from build123d import *

# Parameters (mm, degrees)
EXTRUDE_1_DEPTH     = 32
EXTRUDE_2_DEPTH     = 18
CUT_EXTRUDE_1_DEPTH = 204.283053893
SKETCH_5_W          = 110.763550328
SKETCH_5_H          = 22
CUT_EXTRUDE_2_DEPTH = 6
CUT_EXTRUDE_3_DEPTH = 36
CUT_EXTRUDE_4_DEPTH = 9
SKETCH_7_R          = 6.5
CUT_EXTRUDE_5_DEPTH = 181.357330689
SKETCH_8_W          = 38
SKETCH_8_H          = 7
EXTRUDE_3_DEPTH     = 30.5
EXTRUDE_START       = 14.5
SKETCH_8_3_R        = 9.5
EXTRUDE_4_DEPTH     = 16


with BuildPart() as part:
    # Sketch 1 → Extrude 1 (new, symmetric)
    with BuildSketch(Plane.XY):
        Polygon((0, 0), (-45, 77.942286341), (-28.545517328, 87.442286341), (8.758035362, 22.830637779), (140, 22.830637779), (140, 0), align=None)
    extrude(amount=EXTRUDE_1_DEPTH, both=True)

    # Sketch 2 → Extrude 2 (add)
    with BuildSketch(Plane(origin=(-45, 77.942286341, 0), x_dir=(0.8660254037844364, 0.5000000000000041, 0), z_dir=(-0.500000000000004, 0.8660254037844363, 0))):
        with BuildLine():
            Line((19, 32), (19, -32))
            Line((19, -32), (51, -32))
            ThreePointArc((51, -32), (83, 0), (51, 32))
            Line((51, 32), (19, 32))
        make_face()
    extrude(amount=-EXTRUDE_2_DEPTH)

    # Sketch 4 → Cut-Extrude 1 (cut, through all)
    with BuildSketch(Plane(origin=(-45, 77.942286341, 0), x_dir=(0.8660254037844364, 0.5000000000000041, 0), z_dir=(-0.500000000000004, 0.8660254037844363, 0))):
        Polygon((0, 21), (6, 17.535898385), (6, -17.535898385), (0, -21), align=None)
    extrude(amount=-CUT_EXTRUDE_1_DEPTH, mode=Mode.SUBTRACT)

    # Sketch 5 → Cut-Extrude 2 (cut)
    with BuildSketch(Plane(origin=(-45, 77.942286341, 0), x_dir=(0.8660254037844364, 0.5000000000000041, 0), z_dir=(-0.500000000000004, 0.8660254037844363, 0))):
        with Locations((41.909126347, 0)):
            Rectangle(SKETCH_5_W, SKETCH_5_H)
    extrude(amount=-CUT_EXTRUDE_2_DEPTH, mode=Mode.SUBTRACT)

    # Sketch 6 → Cut-Extrude 3 (cut)
    with BuildSketch(Plane(origin=(-45, 77.942286341, 0), x_dir=(0.8660254037844364, 0.5000000000000041, 0), z_dir=(-0.500000000000004, 0.8660254037844363, 0))):
        with BuildLine():
            ThreePointArc((41.5, 0), (51, -9.5), (60.5, 0))
            Line((60.5, 0), (41.5, 0))
        make_face()
        with BuildLine():
            Line((41.5, 0), (60.5, 0))
            ThreePointArc((60.5, 0), (51, 9.5), (41.5, 0))
        make_face()
    extrude(amount=-CUT_EXTRUDE_3_DEPTH, mode=Mode.SUBTRACT)

    # Sketch 6_3 → Cut-Extrude 4 (cut)
    with BuildSketch(Plane(origin=(-45, 77.942286341, 0), x_dir=(0.8660254037844364, 0.5000000000000041, 0), z_dir=(-0.500000000000004, 0.8660254037844363, 0))):
        with BuildLine():
            ThreePointArc((41.5, 0), (51, -9.5), (60.5, 0))
            Line((60.5, 0), (41.5, 0))
        make_face()
        with BuildLine():
            Line((41.5, 0), (60.5, 0))
            ThreePointArc((60.5, 0), (51, 9.5), (41.5, 0))
        make_face()
        with BuildLine():
            ThreePointArc((41.5, 0), (51, 9.5), (60.5, 0))
            Line((60.5, 0), (67, 0))
            ThreePointArc((67, 0), (65.8644408, 5.92016889), (62.618950039, 11))
            Line((62.618950039, 11), (39.381049961, 11))
            ThreePointArc((39.381049961, 11), (36.1355592, 5.92016889), (35, 0))
            Line((35, 0), (41.5, 0))
        make_face()
        with BuildLine():
            Line((39.381049961, 11), (62.618950039, 11))
            ThreePointArc((62.618950039, 11), (51, 16), (39.381049961, 11))
        make_face()
        with BuildLine():
            Line((67, 0), (60.5, 0))
            ThreePointArc((60.5, 0), (51, -9.5), (41.5, 0))
            Line((41.5, 0), (35, 0))
            ThreePointArc((35, 0), (51, -16), (67, 0))
        make_face()
    extrude(amount=-CUT_EXTRUDE_4_DEPTH, mode=Mode.SUBTRACT)

    # Sketch 7 → Cut-Extrude 5 (cut, through all)
    with BuildSketch(Plane(origin=(5.196152423, 3, 0), x_dir=(0, 0, 1), z_dir=(-0.8660254037844365, -0.500000000000004, 0))):
        with Locations(Location((0, 56, 0), (0, 0, 270))):
            Circle(SKETCH_7_R)
        with Locations(Location((0, 27, 0), (0, 0, 270))):
            Circle(SKETCH_7_R)
    extrude(amount=-CUT_EXTRUDE_5_DEPTH, mode=Mode.SUBTRACT)

    # Sketch 8 → Extrude 3 (add, symmetric)
    with BuildSketch(Plane(origin=(89.5, 0, 0), x_dir=(0, 0, -1), z_dir=(1, 0, 0))):
        with Locations((0, 26.330637779)):
            Rectangle(SKETCH_8_W, SKETCH_8_H)
    extrude(amount=EXTRUDE_3_DEPTH, both=True)

    # Sketch 8_3 → Extrude 4 (add)
    with BuildSketch(Plane(origin=(89.5, 0, 0), x_dir=(0, 0, -1), z_dir=(1, 0, 0)).offset(EXTRUDE_START)):
        with BuildLine():
            Line((-19, 54.830637779), (-19, 29.830637779))
            Line((-19, 29.830637779), (19, 29.830637779))
            Line((19, 29.830637779), (19, 54.830637779))
            ThreePointArc((19, 54.830637779), (0, 73.830637779), (-19, 54.830637779))
        make_face()
        with Locations((0, 54.830637779)):
            Circle(SKETCH_8_3_R, mode=Mode.SUBTRACT)
    extrude_4 = extrude(amount=EXTRUDE_4_DEPTH)

    # Mirror 1: Extrude 4 across plane
    add(extrude_4.mirror(Plane(origin=(89.5, 0, 0), x_dir=(0, 0, 1), z_dir=(1, 0, 0))))


solid = part.part
Work out the finished part from the listing and answer in its coordinate system (mm). A direction names the side the tool comes from. Coordinates: 2 decimals unless noted, no trailing zeros. Write each loop counter-clockwise with the first axis right and the second up, starting at its lowest first coordinate (ties: lowest second). Pieces come first, ordered by that corner, then holes. Notation, with made-up numbers: M -29.75,-28.75 L 3.25,-28.75 A26 cw 3.25,-14.75 Z; hole C 60.5,-14 d11. An arc over 180 degrees is marked long. Use one line per item in the form item = value. Start each with the question number.
1. Each of these flat-tipped pins is pushed along its axis until it touches: P1, Ø11.5, axis at y = 42, z = -7, coming from the -X side; P2, Ø4, axis at x = 13.5, z = -14.5, coming from the +Y side; P3, Ø6, axis at x = 38.5, z = -4, coming from the +Y side. Where does it stop, or does it pass through?
2. Straight lines are drawn through the part: probe 1 along Y at (x, z) = (64.5, 0); probe 2 along X at (y, z) = (41, -15); probe 3 along Z at (x, y) = (-8.5, 93). For each, find the intervals that lie inside material, in ascending order. Write a range as from..to.
3. The part is cut by section A-A (z = -24). Give the vertices of the cut face in (x, y), plus the area to 3 significant figures.
4. The part is cut by section C-C (z = 26). Give the vertices of the cut face in (x, y), plus the area to 3 significant figures.
5. The part is cut by section B-B (y = 10). Give the vertices of the cut face in (x, z), plus the area to 3 significant figures.
6. A tool of negligible diameter and unlimited length cuts with its end or side. For faces 5 (the face through (111.888, 73.826, -0.418)), 6 (the face through (-24, 87, 11)), 7 (the face through (104, 42, 0)), 8 (the face through (90, 28, -19)), 9 (the face through (-16.765, 41.038, -0.246)), from which of +Z, -Z, +X, -X, +Y, -Y can it reach the whole face along a straight path? Write none if from no direction.
7. The mould has two halves that part along X. Classify faces 1 (the face through (19, 111, 11)), 2 (the face through (13.5, 96.2, 3.6)), 3 (the face through (-22.552, 83.975, -0.154)), 4 (the face through (9.63, 99.09, 6.89)): released by +X, released by -X, zero draft, split by the parting line, or undercut.
Evaluation:
q1.P1 = -20.64
q1.P2 = 112.87
q1.P3 = 104.06
q2.probe_1 = 0..45.33, 64.33..73.83
q2.probe_2 = -16.74..-1.73, 59..75, 104..120
q2.probe_3 = -32..-11, 11..32
q3.outline = M -45,77.94 L 0,0 L 140,0 L 140,22.83 L 8.76,22.83 L -19.55,71.85 L 26.5,98.44 L 17.5,114.03 Z
q3.area = 5,620 mm^2
q4.outline = M -45,77.94 L 0,0 L 140,0 L 140,22.83 L 8.76,22.83 L -19.55,71.85 L 24.32,97.18 L 15.32,112.77 Z
q4.area = 5,570 mm^2
q5.outline = M -5.77,-32 L 140,-32 L 140,32 L -5.77,32 L -5.77,21 L 1.15,17.54 L 1.15,-17.54 L -5.77,-21 Z
q5.area = 9,060 mm^2
q6.face_5 = +X, +Y
q6.face_6 = -X, +Y
q6.face_7 = +Z, -Z, +Y
q6.face_8 = -Z, +X, +Y
q6.face_9 = -X, -Y
q7.face_1 = zero draft
q7.face_2 = undercut
q7.face_3 = released by -X
q7.face_4 = undercut
